Read the model definition and answer for the solid it produces. Units are mm, in the model's axes. Coordinates: 2 decimals unless noted, no trailing zeros. Order: outer loops, then holes, each group sorted by start corner. A loop starts at its lowest first (then second) coordinate and runs counter-clockwise, first axis right, second up.
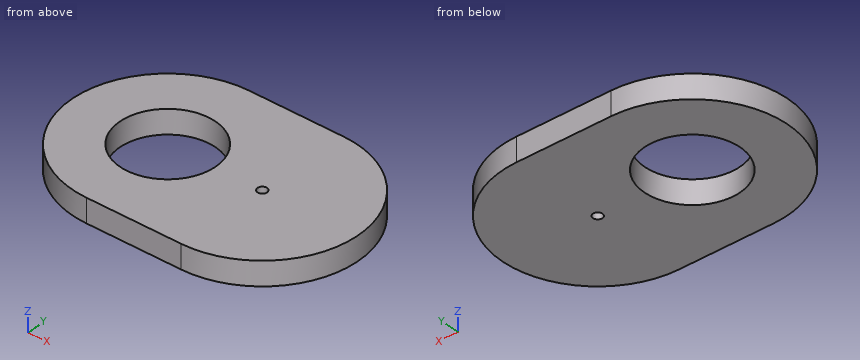
from build123d import *

# Parameters (mm, degrees)
BOSS_EXTRUDE1_DEPTH = 6.35
SKETCH3_6_R         = 12.7
CUT_EXTRUDE1_DEPTH  = 6.35
SKETCH3_9_R         = 1.27
CUT_EXTRUDE5_DEPTH  = 6.35


with BuildPart() as part:
    # Sketch3 → Boss-Extrude1 (new body)
    with BuildSketch(Plane.XY):
        with BuildLine():
            Line((-1.03476248, -23.06540758), (24.36523752, -23.06540758))
            ThreePointArc((24.36523752, -23.06540758), (49.76523752, -48.46540758), (24.36523752, -73.86540758))
            Line((24.36523752, -73.86540758), (-1.03476248, -73.86540758))
            ThreePointArc((-1.03476248, -73.86540758), (-26.43476248, -48.46540758), (-1.03476248, -23.06540758))
        make_face()
    extrude(amount=BOSS_EXTRUDE1_DEPTH)

    # Sketch3<6> → Cut-Extrude1 (cut)
    with BuildSketch(Plane.XY):
        with Locations((-1.03476248, -48.46540758)):
            Circle(SKETCH3_6_R)
    extrude(amount=CUT_EXTRUDE1_DEPTH, mode=Mode.SUBTRACT)

    # Sketch3<9> → Cut-Extrude5 (cut)
    with BuildSketch(Plane.XY):
        with Locations((24.36523752, -48.46540758)):
            Circle(SKETCH3_9_R)
    extrude(amount=CUT_EXTRUDE5_DEPTH, mode=Mode.SUBTRACT)


solid = part.part
Q1. The part is cut by section D-D, the plane y = -29.5. Determine the outline of the cut face in (x, z).
Q2. The part is cut by section C-C, the plane z = 3.25. Determine the outline of the cut face in (x, y).
Q3. The part is cut by section A-A, the plane x = -5. Determine the outline of the cut face in (y, z).
Q4. Each of these flat-tipped pins is pushed along its axis until it touches: P1, Ø2, axis at y = -54, z = 2, coming from the -X side; P2, Ø1.5, axis at x = -12, z = 4, coming from the -Y side; P3, Ø3, axis at x = -16.5, z = 5, coming from the -Y side. Where does it stop, or does it pass through?
Q5. Straight lines are drawn through the part: L1, parallel to Y at x = 0, z = 5.25; L2, parallel to X at y = -48, z = 1.25; L3, parallel to Y at x = -2, z = 5. For each, find the intervals that lie inside material, in ascending order.
Q6. The part is cut by section B-B, the plane y = -37. Determine the outline of the cut face in (x, z).
Computed values:
1. outline: (-17.93, 0) - (41.26, 0) - (41.26, 6.35) - (-17.93, 6.35) - close
2. outline: (-1.03, -73.87) - (24.37, -73.87) arc R25.4 ccw to (24.37, -23.07) - (-1.03, -23.07) arc R25.4 ccw to start; hole circle Ø25.4 at (-1.03, -48.47); hole circle Ø2.54 at (24.37, -48.47)
3. outline: (-73.55, 0) - (-60.53, 0) - (-60.53, 6.35) - (-73.55, 6.35) - close; (-36.4, 0) - (-23.38, 0) - (-23.38, 6.35) - (-36.4, 6.35) - close
4. P1: stops at x = -26.03
4. P2: stops at y = -71.72
4. P3: stops at y = -69.68
5. L1: y = -73.87 to -61.12, -35.81 to -23.07
5. L2: x = -26.43 to -13.73, 11.66 to 23.18, 25.55 to 49.76
5. L3: y = -73.85 to -61.13, -35.8 to -23.08
6. outline: (-23.7, 0) - (-6.5, 0) - (-6.5, 6.35) - (-23.7, 6.35) - close; (4.43, 0) - (47.03, 0) - (47.03, 6.35) - (4.43, 6.35) - close
